from build123d import *

# Parameters (mm, degrees)
EXTRUDE_1_DEPTH          = 240
EXTRUDE_2_DEPTH          = 35
EXTRUDE_3_DEPTH          = 35
EXTRUDE_5_DEPTH          = 35
EXTRUDE_5_DEPTH_BACK     = 90
SKETCH_9_W               = 90
SKETCH_9_H               = 110
SKETCH_10_R              = 65
CUT_EXTRUDE_1_DEPTH      = 389.72387372
CUT_EXTRUDE_2_REACH      = 416.427
CUT_EXTRUDE_2_END_RADIUS = 65
SKETCH_12_R              = 35
CUT_EXTRUDE_3_REACH      = 437.448
SKETCH_15_R              = 10
SKETCH_16_R              = 5
CUT_EXTRUDE_4_DEPTH      = 30
FILLET_13_R              = 10
FILLET_15_R              = 10


with BuildPart() as part:
    # Эскиз1 → Бобышка-Вытянуть1 (new body)
    with BuildSketch(Plane.XY):
        Polygon((0, 103.923048454), (-90, 51.961524227), (-90, -51.961524227), (-22.5, -90.932667397), (-22.5, -145), (-107.5, -145), (-107.5, -190), (107.5, -190), (107.5, -145), (22.5, -145), (22.5, -90.932667397), (90, -51.961524227), (90, 51.961524227), align=None)
    extrude(amount=EXTRUDE_1_DEPTH)

    # Эскиз2 → Бобышка-Вытянуть2 (add)
    with BuildSketch(Plane.XY.offset(240)):
        Polygon((0, 118.356805184), (-102.5, 59.178402592), (-102.5, -59.178402592), (0, -118.356805184), (102.5, -59.178402592), (102.5, 59.178402592), align=None)
    extrude(amount=EXTRUDE_2_DEPTH)

    # Эскиз6 → Бобышка-Вытянуть3 (add)
    with BuildSketch(Plane(origin=(0, 0, 0), x_dir=(-1, 0, 0), z_dir=(0, 0, -1))):
        Polygon((0, 118.356805184), (-102.5, 59.178402592), (-102.5, -59.178402592), (0, -118.356805184), (102.5, -59.178402592), (102.5, 59.178402592), align=None)
    extrude(amount=EXTRUDE_3_DEPTH)

    # Эскиз9 → Бобышка-Вытянуть5 (add, two sides: drawn at the far end of the back side and taken through both)
    with BuildSketch(Plane(origin=(102.5, 0, 0), x_dir=(0, 0, -1), z_dir=(1, 0, 0)).offset(-EXTRUDE_5_DEPTH_BACK)):
        with Locations((-85, 5)):
            Rectangle(SKETCH_9_W, SKETCH_9_H)
    extrude(amount=EXTRUDE_5_DEPTH + EXTRUDE_5_DEPTH_BACK)

    # Эскиз10 → Вырез-Вытянуть1 (cut, through all)
    with BuildSketch(Plane.XY.offset(275)):
        Circle(SKETCH_10_R)
    extrude(amount=-CUT_EXTRUDE_1_DEPTH, mode=Mode.SUBTRACT)

    # Вырез-Вытянуть2: up to this cylinder (the profile starts outside it)
    cut_extrude_2_end = Plane(origin=(0, 0, 85.10225), z_dir=(0, 0, 1)) * Cylinder(CUT_EXTRUDE_2_END_RADIUS, 963.854, mode=Mode.PRIVATE)
    # Эскиз12 → Вырез-Вытянуть2 (cut, up to the surface)
    with BuildSketch(Plane(origin=(137.5, 0, 0), x_dir=(0, 0, -1), z_dir=(1, 0, 0)), mode=Mode.PRIVATE) as cut_extrude_2_sk1:
        with Locations(Location((-85.102250197, 4.574709124, 0), (0, 0, 90))):
            Circle(SKETCH_12_R)
    cut_extrude_2_tool1 = extrude(cut_extrude_2_sk1.sketch, amount=-CUT_EXTRUDE_2_REACH, mode=Mode.PRIVATE) - cut_extrude_2_end
    add(cut_extrude_2_tool1.solids().sort_by_distance((137.5, 4.574709, 85.10225))[0], mode=Mode.SUBTRACT)

    # Эскиз15 → Вырез-Вытянуть3 (cut, up to next)
    with BuildSketch(Plane(origin=(0, -190, 0), x_dir=(-1, 0, 0), z_dir=(0, -1, 0)), mode=Mode.PRIVATE) as cut_extrude_3_sk1:
        with Locations(Location((87.5, -220, 0), (0, 0, 90))):
            Circle(SKETCH_15_R)
    cut_extrude_3_tool1 = extrude(cut_extrude_3_sk1.sketch, amount=-CUT_EXTRUDE_3_REACH, mode=Mode.PRIVATE) & part.part
    # Эскиз15 → Вырез-Вытянуть3 (cut, up to next)
    with BuildSketch(Plane(origin=(0, -190, 0), x_dir=(-1, 0, 0), z_dir=(0, -1, 0)), mode=Mode.PRIVATE) as cut_extrude_3_sk2:
        with Locations(Location((-87.5, -220, 0), (0, 0, 90))):
            Circle(SKETCH_15_R)
    cut_extrude_3_tool2 = extrude(cut_extrude_3_sk2.sketch, amount=-CUT_EXTRUDE_3_REACH, mode=Mode.PRIVATE) & part.part
    # Эскиз15 → Вырез-Вытянуть3 (cut, up to next)
    with BuildSketch(Plane(origin=(0, -190, 0), x_dir=(-1, 0, 0), z_dir=(0, -1, 0)), mode=Mode.PRIVATE) as cut_extrude_3_sk3:
        with Locations(Location((-87.5, -20, 0), (0, 0, 90))):
            Circle(SKETCH_15_R)
    cut_extrude_3_tool3 = extrude(cut_extrude_3_sk3.sketch, amount=-CUT_EXTRUDE_3_REACH, mode=Mode.PRIVATE) & part.part
    # Эскиз15 → Вырез-Вытянуть3 (cut, up to next)
    with BuildSketch(Plane(origin=(0, -190, 0), x_dir=(-1, 0, 0), z_dir=(0, -1, 0)), mode=Mode.PRIVATE) as cut_extrude_3_sk4:
        with Locations(Location((87.5, -20, 0), (0, 0, 90))):
            Circle(SKETCH_15_R)
    cut_extrude_3_tool4 = extrude(cut_extrude_3_sk4.sketch, amount=-CUT_EXTRUDE_3_REACH, mode=Mode.PRIVATE) & part.part
    add(cut_extrude_3_tool1.solids().sort_by_distance((-87.5, -190, 220))[0], mode=Mode.SUBTRACT)
    add(cut_extrude_3_tool2.solids().sort_by_distance((87.5, -190, 220))[0], mode=Mode.SUBTRACT)
    add(cut_extrude_3_tool3.solids().sort_by_distance((87.5, -190, 20))[0], mode=Mode.SUBTRACT)
    add(cut_extrude_3_tool4.solids().sort_by_distance((-87.5, -190, 20))[0], mode=Mode.SUBTRACT)

    # Эскиз16 → Вырез-Вытянуть4 (cut)
    with BuildSketch(Plane(origin=(137.5, 0, 0), x_dir=(0, 0, -1), z_dir=(1, 0, 0))):
        with Locations(Location((-120, 50, 0), (0, 0, 90))):
            Circle(SKETCH_16_R)
        with Locations(Location((-50, 50, 0), (0, 0, 90))):
            Circle(SKETCH_16_R)
        with Locations(Location((-120, -40, 0), (0, 0, 90))):
            Circle(SKETCH_16_R)
        with Locations(Location((-50, -40, 0), (0, 0, 90))):
            Circle(SKETCH_16_R)
    extrude(amount=-CUT_EXTRUDE_4_DEPTH, mode=Mode.SUBTRACT)

    # Скругление13
    # the kernel refuses this fillet: 10 mm, written as the material it takes off along each edge
    with BuildSketch(Plane(origin=(51.076951546, 60, 40), x_dir=(0, 0, 1), z_dir=(1, 0, 0))) as fillet_13_piece_1_section:
        with BuildLine():
            CenterArc((FILLET_13_R, FILLET_13_R), FILLET_13_R, 180, 90)
            Line((0, FILLET_13_R), (0, 0))
            Line((0, 0), (FILLET_13_R, 0))
        make_face()
    fillet_13_piece_1 = extrude(amount=111.423048454, mode=Mode.PRIVATE)
    fillet_13_piece_1 = split(fillet_13_piece_1, bisect_by=Plane(origin=(91.336979789, 51.189618586, 39.919231597), z_dir=(-0.5000000000000002, -0.8660254037844386, 0)), keep=Keep.TOP, mode=Mode.PRIVATE)
    fillet_13_piece_1 = split(fillet_13_piece_1, bisect_by=Plane(origin=(90, 50.726475201, 39.919231597), z_dir=(1, 0, 0)), keep=Keep.TOP, mode=Mode.PRIVATE)
    add(fillet_13_piece_1, mode=Mode.SUBTRACT)
    with BuildSketch(Plane(origin=(51.076951546, 60, 40), x_dir=(0, 0, 1), z_dir=(1, 0, 0))) as fillet_13_piece_2_section:
        with BuildLine():
            CenterArc((FILLET_13_R, FILLET_13_R), FILLET_13_R, 180, 90)
            Line((0, FILLET_13_R), (0, 0))
            Line((0, 0), (FILLET_13_R, 0))
        make_face()
    fillet_13_piece_2 = extrude(amount=111.423048454, mode=Mode.PRIVATE)
    fillet_13_piece_2 = split(fillet_13_piece_2, bisect_by=Plane(origin=(82.903194499, 56.058866794, 42.730902083), z_dir=(0.5000000000000002, 0.8660254037844386, 0)), keep=Keep.TOP, mode=Mode.PRIVATE)
    fillet_13_piece_2 = split(fillet_13_piece_2, bisect_by=Plane(origin=(90, 58.517272333, 42.730902083), z_dir=(-1, 0, 0)), keep=Keep.TOP, mode=Mode.PRIVATE)
    add(fillet_13_piece_2, mode=Mode.SUBTRACT)
    with BuildSketch(Plane(origin=(51.076951546, 60, 40), x_dir=(0, 0, 1), z_dir=(1, 0, 0))) as fillet_13_piece_3_section:
        with BuildLine():
            CenterArc((FILLET_13_R, FILLET_13_R), FILLET_13_R, 180, 90)
            Line((0, FILLET_13_R), (0, 0))
            Line((0, 0), (FILLET_13_R, 0))
        make_face()
    fillet_13_piece_3 = extrude(amount=111.423048454, mode=Mode.PRIVATE)
    fillet_13_piece_3 = split(fillet_13_piece_3, bisect_by=Plane(origin=(114.69683315, 37.70280096, 42.264932775), z_dir=(0.5000000000000002, 0.8660254037844386, 0)), keep=Keep.TOP, mode=Mode.PRIVATE)
    fillet_13_piece_3 = split(fillet_13_piece_3, bisect_by=Plane(origin=(90, 57.738983461, 42.264932775), z_dir=(1, 0, 0)), keep=Keep.TOP, mode=Mode.PRIVATE)
    add(fillet_13_piece_3, mode=Mode.SUBTRACT)
    with BuildSketch(Plane(origin=(162.5, 60, 130), x_dir=(0, -1, 0), z_dir=(-1, 0, 0))) as fillet_13_piece_4_section:
        with BuildLine():
            CenterArc((FILLET_13_R, -FILLET_13_R), FILLET_13_R, 90, 90)
            Line((0, -FILLET_13_R), (0, 0))
            Line((0, 0), (FILLET_13_R, 0))
        make_face()
    fillet_13_piece_4 = extrude(amount=111.423048454, mode=Mode.PRIVATE)
    fillet_13_piece_4 = split(fillet_13_piece_4, bisect_by=Plane(origin=(114.69683315, 37.70280096, 127.735067225), z_dir=(0.5000000000000002, 0.8660254037844386, 0)), keep=Keep.TOP, mode=Mode.PRIVATE)
    fillet_13_piece_4 = split(fillet_13_piece_4, bisect_by=Plane(origin=(90, 57.738983461, 127.735067225), z_dir=(1, 0, 0)), keep=Keep.TOP, mode=Mode.PRIVATE)
    add(fillet_13_piece_4, mode=Mode.SUBTRACT)
    with BuildSketch(Plane(origin=(162.5, 60, 130), x_dir=(0, -1, 0), z_dir=(-1, 0, 0))) as fillet_13_piece_5_section:
        with BuildLine():
            CenterArc((FILLET_13_R, -FILLET_13_R), FILLET_13_R, 90, 90)
            Line((0, -FILLET_13_R), (0, 0))
            Line((0, 0), (FILLET_13_R, 0))
        make_face()
    fillet_13_piece_5 = extrude(amount=111.423048454, mode=Mode.PRIVATE)
    fillet_13_piece_5 = split(fillet_13_piece_5, bisect_by=Plane(origin=(82.903194499, 56.058866793, 127.269097917), z_dir=(0.5000000000000002, 0.8660254037844386, 0)), keep=Keep.TOP, mode=Mode.PRIVATE)
    fillet_13_piece_5 = split(fillet_13_piece_5, bisect_by=Plane(origin=(90, 58.517272333, 127.269097917), z_dir=(-1, 0, 0)), keep=Keep.TOP, mode=Mode.PRIVATE)
    add(fillet_13_piece_5, mode=Mode.SUBTRACT)
    with BuildSketch(Plane(origin=(162.5, 60, 130), x_dir=(0, -1, 0), z_dir=(-1, 0, 0))) as fillet_13_piece_6_section:
        with BuildLine():
            CenterArc((FILLET_13_R, -FILLET_13_R), FILLET_13_R, 90, 90)
            Line((0, -FILLET_13_R), (0, 0))
            Line((0, 0), (FILLET_13_R, 0))
        make_face()
    fillet_13_piece_6 = extrude(amount=111.423048454, mode=Mode.PRIVATE)
    fillet_13_piece_6 = split(fillet_13_piece_6, bisect_by=Plane(origin=(91.336979789, 51.189618586, 130.080768403), z_dir=(-0.5000000000000002, -0.8660254037844386, 0)), keep=Keep.TOP, mode=Mode.PRIVATE)
    fillet_13_piece_6 = split(fillet_13_piece_6, bisect_by=Plane(origin=(90, 50.726475201, 130.080768403), z_dir=(1, 0, 0)), keep=Keep.TOP, mode=Mode.PRIVATE)
    add(fillet_13_piece_6, mode=Mode.SUBTRACT)
    with BuildSketch(Plane(origin=(90, -50, 40), x_dir=(0, 1, 0), z_dir=(1, 0, 0)), Plane(origin=(162.5, -50, 130), x_dir=(0, 1, 0), z_dir=(-1, 0, 0))) as fillet_13_piece_7:
        with BuildLine():
            CenterArc((FILLET_13_R, FILLET_13_R), FILLET_13_R, 180, 90)
            Line((0, FILLET_13_R), (0, 0))
            Line((0, 0), (FILLET_13_R, 0))
        make_face()
    extrude(amount=72.5, mode=Mode.SUBTRACT)

    # Скругление15
    fillet_15_edges = [part.edges().sort_by_distance(p)[0] for p in [
        (107.5, -167.5, 0),
        (-107.5, -167.5, 0),
        (-107.5, -167.5, 240),
        (107.5, -167.5, 240),
    ]]
    fillet(fillet_15_edges, radius=FILLET_15_R)


solid = part.part
Design review of the part built by this model. Coordinates are the model's own, in mm. A direction names the side the tool comes from. Round coordinates to 2 decimals unless told otherwise and drop trailing zeros. Order: outer loops, then holes, each group sorted by start corner. A loop starts at its lowest first (then second) coordinate and runs counter-clockwise, first axis right, second up.
1) Consider section A-A (z = 20). State the section outline as (x, y) points.
The answers:
outline: (-107.5, -190) - (-97.5, -190) - (-97.5, -145) - (-107.5, -145) - close; (-90, -51.96) - (-22.5, -90.93) - (-22.5, -145) - (-77.5, -145) - (-77.5, -190) - (77.5, -190) - (77.5, -145) - (22.5, -145) - (22.5, -90.93) - (90, -51.96) - (90, 51.96) - (0, 103.92) - (-90, 51.96) - close; (97.5, -190) - (107.5, -190) - (107.5, -145) - (97.5, -145) - close; hole circle Ø130 at (0, 0)
2) Consider section B-B (y = -12). State the section outline as (x, z) points, plus the area to 3 significant figures.
The answers:
outline: (-102.5, -35) - (-63.88, -35) - (-63.88, 275) - (-102.5, 275) - (-102.5, 240) - (-90, 240) - (-90, 0) - (-102.5, 0) - close; (63.88, -35) - (102.5, -35) - (102.5, 0) - (90, 0) - (90, 40) - (137.5, 40) - (137.5, 54.28) - (63.88, 54.28) - close; (63.88, 115.93) - (137.5, 115.93) - (137.5, 130) - (90, 130) - (90, 240) - (102.5, 240) - (102.5, 275) - (63.88, 275) - close
area: 17,700 mm2
3) Machinability: for faces 1 (the flat face through (54, 73, 0)), 2 (the cylindrical face through (95.93, -167.82, 214.62)), 3 (the flat face through (113, -50, 85)), which of the approach directions +Z, -Z, +X, -X, +Y, -Y give a long, thin tool a straight path to every point of the face, cutting with its end or side? Answer none if there is none.
The answers:
face 1: none
face 2: -Y
face 3: +X
4) Consider section C-C (x = 47). State the section outline as (y, z) points, plus the area to 3 significant figures.
The answers:
outline: (-190, 0) - (-145, 0) - (-145, 240) - (-190, 240) - close; (-91.22, -35) - (-44.9, -35) - (-44.9, 275) - (-91.22, 275) - (-91.22, 240) - (-76.79, 240) - (-76.79, 0) - (-91.22, 0) - close; (44.9, -35) - (91.22, -35) - (91.22, 0) - (76.79, 0) - (76.79, 240) - (91.22, 240) - (91.22, 275) - (44.9, 275) - close
area: 32,600 mm2
5) For L1, parallel to Z at x = 117, y = 50; L2, parallel to X at y = -162, z = 220; L3, parallel to Z at x = 80, y = -67.5, list the stretches that pass through material, from the lowest coordinate up.
The answers:
L1: z = 40 to 45, 55 to 115, 125 to 130
L2: x = -107.5 to -97.5, -77.5 to 77.5, 97.5 to 107.5
L3: z = -35 to 0, 240 to 275
6) Clearance check with flat-ended pins moving along their axes: pin 1 Ø8 at (y, z) = (-39, 119.5) entering from +X; pin 2 Ø10.5 at (y, z) = (-15, 264.5) entering from -X; pin 3 Ø10.5 at (y, z) = (-6.5, -9.5) entering from +X; pin 4 Ø6 at (y, z) = (1.5, 205.5) entering from +X. State where each tip first meets the part, or that it passes through.
The answers:
pin 1: stops at x = 137.5
pin 2: stops at x = -102.5
pin 3: stops at x = 102.5
pin 4: stops at x = 90
7) Draft analysis for pull direction Y (two halves, no side actions). For faces 4 (the flat face through (102.5, 1, -17)), 5 (the cylindrical face through (122.71, 49.349, 54.957)), 6 (the flat face through (-2, -190, 118)), 7 (the flat face through (107.5, 50, 50)), state which applies: released by +Y, released by -Y, zero draft, split by the parting line, or undercut.
The answers:
face 4: zero draft
face 5: undercut
face 6: released by -Y
face 7: undercut
8) Consider section D-D (z = 159). State the section outline as (x, y) points.
The answers:
outline: (-107.5, -190) - (107.5, -190) - (107.5, -145) - (22.5, -145) - (22.5, -90.93) - (90, -51.96) - (90, 51.96) - (0, 103.92) - (-90, 51.96) - (-90, -51.96) - (-22.5, -90.93) - (-22.5, -145) - (-107.5, -145) - close; hole circle Ø130 at (0, 0)
